Geometry check sheet. Reference: the model listing, model coordinates, mm. Coordinates: 2 decimals unless noted, no trailing zeros. Write each loop counter-clockwise with the first axis right and the second up, starting at its lowest first coordinate (ties: lowest second). Pieces come first, ordered by that corner, then holes.
from build123d import *

# Parameters (mm, degrees)
PAD_DEPTH     = 3
SKETCH001_R   = 1
SKETCH001_R_2 = 2.1
POCKET_DEPTH  = 3


with BuildPart() as part:
    # Sketch → Pad (new body)
    with BuildSketch(Plane.XY):
        with BuildLine():
            ThreePointArc((-39.153312, -17), (0, -23.9385), (39.153312, -17))
            ThreePointArc((39.153312, -17), (47.135393, 12.608816), (17.853572, 3.5))
            ThreePointArc((-17.853572, 3.5), (0, -9.681542), (17.853572, 3.5))
            ThreePointArc((-17.853572, 3.5), (-47.135393, 12.608816), (-39.153312, -17))
        make_face()
    extrude(amount=PAD_DEPTH)

    # Sketch001 (on Face6 of Pad) → Pocket (cut)
    with BuildSketch(Plane.XY.offset(3)):
        with Locations((-35, 11)):
            Circle(SKETCH001_R)
        with Locations((-35, -11)):
            Circle(SKETCH001_R)
        with Locations((-46, 0)):
            Circle(SKETCH001_R)
        with Locations((-24, 0)):
            Circle(SKETCH001_R)
        with Locations((-35, 0)):
            Circle(SKETCH001_R_2)
    pocket = extrude(amount=-POCKET_DEPTH, mode=Mode.SUBTRACT)

    # Mirrored: Pocket across Sketch001 V_Axis
    add(pocket.mirror(Plane(origin=(0, 0, 3), x_dir=(0, 0, 1), z_dir=(1, 0, 0))), mode=Mode.SUBTRACT)


solid = part.part
1. Sectioned sample at D-D, the plane x = 46. Record the boundary of the cut face in (y, z), and give its area (3 significant figures).
Computed values:
outline: (-13.61, 0) - (-1, 0) - (-1, 3) - (-13.61, 3) - close; (1, 0) - (13.61, 0) - (13.61, 3) - (1, 3) - close
area: 75.7 mm2
2. Sectioned sample at A-A, the plane z = 2.1. Give the number of separate pieces and of enclosed holes in the cut face, and give its area (3 significant figures).
Computed values:
separate pieces: 1
enclosed holes: 10
area: 2,720 mm2
3. Gauge pin test, flat ends, axial feed: pin 1 Ø12 at (x, y) = (18.5, -3.5) entering from -Z; pin 2 Ø1 at (x, z) = (30.5, 1) entering from -Y. Record the tip position at first contact, or that the pin passes through.
Computed values:
pin 1: stops at z = 0
pin 2: stops at y = -19.92
4. Draft check along Y on faces 1 (the flat face through (-1, -12, 0)), 2 (the cylindrical face through (-46.75, 12.97, 1.48)), 3 (the cylindrical face through (-45, 0, 2)). Enter one of: released by +Y, released by -Y, zero draft, split by the parting line, or undercut.
Computed values:
face 1: zero draft
face 2: split by the parting line
face 3: undercut
5. Sectioned sample at B-B, the plane y = 6. Record the boundary of the cut face in (x, z), and give its area (3 significant figures).
Computed values:
outline: (-51.44, 0) - (-18.56, 0) - (-18.56, 3) - (-51.44, 3) - close; (18.56, 0) - (51.44, 0) - (51.44, 3) - (18.56, 3) - close
area: 197 mm2
6. Thickness scan on line 1 along Y through (x, z) = (-35, 2.15); line 2 along Y through (x, z) = (-46, 2.2); line 3 along X through (y, z) = (15, 0.55). Record the ranges inside material, lowest first.
Computed values:
line 1: y = -18.43 to -12, -10 to -2.1, 2.1 to 10, 12 to 17.5
line 2: y = -13.61 to -1, 1 to 13.61
line 3: x = -44.01 to -25.99, 25.99 to 44.01
7. Sectioned sample at C-C, the plane x = -35. Record the boundary of the cut face in (y, z), and give its area (3 significant figures).
Computed values:
outline: (-18.43, 0) - (-12, 0) - (-12, 3) - (-18.43, 3) - close; (-10, 0) - (-2.1, 0) - (-2.1, 3) - (-10, 3) - close; (2.1, 0) - (10, 0) - (10, 3) - (2.1, 3) - close; (12, 0) - (17.5, 0) - (17.5, 3) - (12, 3) - close
area: 83.2 mm2
